Source: CAD feature listing. Evaluate the final solid. Frame: model axes, mm. A direction names the side the tool comes from. Give positions to 0.01 mm unless a question says otherwise; leave off trailing zeros. Write each loop counter-clockwise with the first axis right and the second up, starting at its lowest first coordinate (ties: lowest second). Pieces come first, ordered by that corner, then holes. Notation, with made-up numbers: M 55.25,-13 L 82.25,-13 A26 ccw 82.25,23 Z; hole C 80.25,5.5 d10. An arc over 180 degrees is marked long. Return JSON: item names as keys, results as strings.
```python
from build123d import *

# Parameters (mm, degrees)
SKETCH2_W           = 77
SKETCH2_H           = 62
BOSS_EXTRUDE1_DEPTH = 2
SKETCH3_W           = 8
SKETCH3_H           = 2
SKETCH3_W_2         = 2
SKETCH3_H_2         = 20
BOSS_EXTRUDE2_DEPTH = 10
SKETCH4_R           = 1.25
CUT_EXTRUDE1_DEPTH  = 63
CUT_EXTRUDE2_REACH  = 79
SKETCH5_R           = 1.25


with BuildPart() as part:
    # Sketch2 → Boss-Extrude1 (new body)
    with BuildSketch(Plane(origin=(0, 0, 0), x_dir=(1, 0, 0), z_dir=(0, 1, 0))):
        with Locations((-4.195246224, 15.849517589)):
            Rectangle(SKETCH2_W, SKETCH2_H)
    extrude(amount=BOSS_EXTRUDE1_DEPTH)

    # Sketch3 → Boss-Extrude2 (add)
    with BuildSketch(Plane(origin=(0, 2, 0), x_dir=(1, 0, 0), z_dir=(0, 1, 0))):
        with Locations((-38.695246224, -14.150482411)):
            Rectangle(SKETCH3_W, SKETCH3_H)
        with Locations((-38.695246224, 45.849517589)):
            Rectangle(SKETCH3_W, SKETCH3_H)
        with Locations((33.304753776, 36.849517589)):
            Rectangle(SKETCH3_W_2, SKETCH3_H_2)
        with Locations((33.304753776, -5.150482411)):
            Rectangle(SKETCH3_W_2, SKETCH3_H_2)
    extrude(amount=BOSS_EXTRUDE2_DEPTH)

    # Sketch4 → Cut-Extrude1 (cut, through all)
    with BuildSketch(Plane.XY.offset(15.150482411)):
        with Locations((-38.695246224, 7)):
            Circle(SKETCH4_R)
    extrude(amount=-CUT_EXTRUDE1_DEPTH, mode=Mode.SUBTRACT)

    # Sketch5 → Cut-Extrude2 (cut, up to next)
    with BuildSketch(Plane(origin=(34.304753776, 0, 0), x_dir=(0, 0, -1), z_dir=(1, 0, 0)), mode=Mode.PRIVATE) as cut_extrude2_sk1:
        with Locations((-3.150482411, 7)):
            Circle(SKETCH5_R)
    cut_extrude2_tool1 = extrude(cut_extrude2_sk1.sketch, amount=-CUT_EXTRUDE2_REACH, mode=Mode.PRIVATE) & part.part
    add(cut_extrude2_tool1.solids().sort_by_distance((34.304754, 7, 3.150482))[0], mode=Mode.SUBTRACT)
    # Sketch5 → Cut-Extrude2 (cut, up to next)
    with BuildSketch(Plane(origin=(34.304753776, 0, 0), x_dir=(0, 0, -1), z_dir=(1, 0, 0)), mode=Mode.PRIVATE) as cut_extrude2_sk2:
        with Locations((34.849517589, 7)):
            Circle(SKETCH5_R)
    cut_extrude2_tool2 = extrude(cut_extrude2_sk2.sketch, amount=-CUT_EXTRUDE2_REACH, mode=Mode.PRIVATE) & part.part
    add(cut_extrude2_tool2.solids().sort_by_distance((34.304754, 7, -34.849518))[0], mode=Mode.SUBTRACT)


solid = part.part
```
1) Cut plane C-C, the plane z = -2. Return the cut outline in (x, y).
Numbers:
{"outline": "M -42.7,0 L 34.3,0 L 34.3,12 L 32.3,12 L 32.3,2 L -42.7,2 Z"}
2) Cut plane B-B, the plane x = -13. Return the cut outline in (y, z).
Numbers:
{"outline": "M 0,-46.85 L 2,-46.85 L 2,15.15 L 0,15.15 Z"}
3) Line query: line 1 (Z direction, x = -39, y = 4.25); line 2 (Y direction, x = -5, z = -41); line 3 (X direction, y = 6.5, z = 7). Output: solid intervals per line, ascending. Write a range as [from, to].
Numbers:
{"line 1": "z = [-46.85, -44.85], [13.15, 15.15]", "line 2": "y = [0, 2]", "line 3": "x = [32.3, 34.3]"}
4) Set-up query: faces 5 (the face through (33, 7, -26.85)), 6 (the face through (-34.695, 7, -46)), 7 (the face through (-37.9, 5.8, 13.15)). Return all of +Z, -Z, +X, -X, +Y, -Y with unobstructed straight access to the full face (end or side cutting, diameter ignored); none if empty.
Numbers:
{"face 5": "+X, -X, +Y", "face 6": "+Z, -Z, +Y", "face 7": "-X, +Y"}
5) Draft query along X for faces 1 (the face through (-5, 0, -16)), 2 (the face through (-42.695, 1.5, -15.7)), 3 (the face through (34.305, 1, -15)), 4 (the face through (-34.695, 7, 14)). Return one class per face: released by +X, released by -X, zero draft, split by the parting line, or undercut.
Numbers:
{"face 1": "zero draft", "face 2": "released by -X", "face 3": "released by +X", "face 4": "undercut"}
6) Contact query for a flat-ended pin moving along its axis: pin 1 Ø3 at (y, z) = (9.5, 5.5) entering from -X. Output: stop coordinate, or through.
Numbers:
{"pin 1": "stops at x = 32.3"}
7) Cut plane D-D, the plane z = -14.5. Return the cut outline in (x, y).
Numbers:
{"outline": "M -42.7,0 L 34.3,0 L 34.3,2 L -42.7,2 Z"}
8) Cut plane A-A, the plane y = 7. Give the number of separate pieces and of enclosed holes in the cut face, then the cut area to 3 significant figures.
Numbers:
{"separate pieces": "8", "enclosed holes": "0", "area": "92.0 mm²"}
